Autodesk Inventor part; units mm, degrees
ref_plane "YZ Plane" through (0, 0, 0) normal (1, 0, 0) x (0, 1, 0)
ref_plane "XZ Plane" through (0, 0, 0) normal (0, 1, 0) x (-1, 0, 0)
ref_plane "XY Plane" through (0, 0, 0) normal (0, 0, 1) x (1, 0, 0)
sketch "Sketch1" plane through (0, 0, 0) normal (0, 1, 0) x (-1, 0, 0)
  line L0 (0, 0) -> (5.4973, 0)
  line L1 (5.4973, 0) -> (5.4973, -16.0791)
  line L2 (5.4973, -16.0791) -> (0, -16.0791)
  line L3 (0, -16.0791) -> (0, 0)
extrude "Extrusion1" add sketch "Sketch1" along normal blind 25.4
sketch "Sketch2" plane through (0, 0, 0) normal (1, 0, 0) x (0, 0, -1)
  line L0 (5.242, 8.6906) -> (11.0751, 8.6906)
  line L1 (11.0751, 8.6906) -> (11.0751, 5.3799)
  line L2 (11.0751, 5.3799) -> (5.242, 5.3799)
  line L3 (5.242, 5.3799) -> (5.242, 8.6906)
  line L4 (12.2594, 20.9027) -> (3.9371, 20.9027)
  line L5 (3.9371, 20.9027) -> (3.9371, 16.3797)
  line L6 (3.9371, 16.3797) -> (12.2594, 16.3797)
  line L7 (12.2594, 16.3797) -> (12.2594, 20.9027)
  point P0 (0, 0)
extrude "Extrusion2" add sketch "Sketch2" along normal blind 5
sketch "Sketch3" plane through (0, 25.4, 0) normal (0, 1, 0) x (1, 0, 0)
  point P0 (0, 0)
sketch "Sketch4" plane through (0, 16.3797, -12.2594) normal (0, 0, -1) x (-1, 0, 0)
  circle A0 centre (-2.546, 2.7504) radius 1.0051
  circle A1 centre (-2.546, -8.9893) radius 0.8063
  point P0 (0, -16.3797)
extrude "Extrusion3" add sketch "Sketch4" along normal blind 15 contours A0
sketch "Sketch5" plane through (0, 5.3799, -11.0751) normal (0, 0, -1) x (-1, 0, 0)
  circle A0 centre (-2.6874, 1.7983) radius 0.9619
  point P0 (0, -5.3799)
extrude "Extrusion4" add sketch "Sketch5" along normal blind 25
properties part number "niharika1"
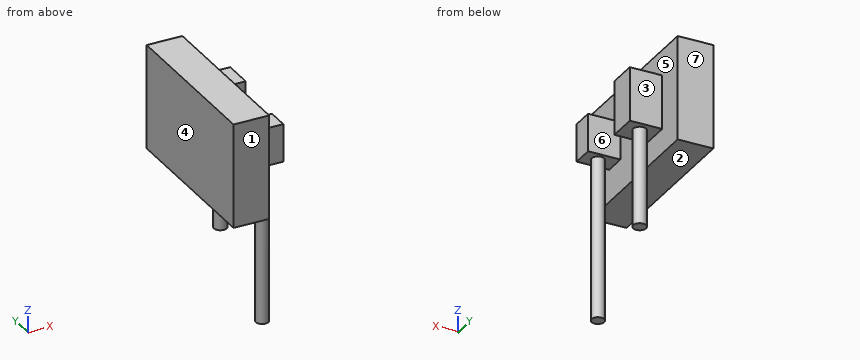
Verification items for the finished model (mm, model axes). Face numbers are marked on the shaded views. A direction names the side the tool comes from. Round coordinates to 2 decimals unless told otherwise and drop trailing zeros. Loops run counter-clockwise (first coordinate to the right, second up) from the corner with the lowest first, then second, coordinate; pieces in that order, holes last. Notation, with made-up numbers: (59, 72.25) -> (72, 72.25) arc R7 cw to (72, 80.25) -> close; hole circle Ø5 at (48.5, 55.25). An arc over 180 degrees is marked (long way). Answer as a JSON object with one key per item and string values.
Q1. Draft check along Y on the marked faces 4, 5, 6 and 7. Enter one of: pulls with the +Y half, pulls with the -Y half, needs draft (parallel to the pull), parting line crosses it, or undercut.
Data:
{"face 4": "needs draft", "face 5": "undercut", "face 6": "undercut", "face 7": "pulls with the +Y half"}
Q2. Section check D-D (x = -2.25). Record the boundary of the cut face in (y, z).
Data:
{"outline": "(0, -16.08) -> (25.4, -16.08) -> (25.4, 0) -> (0, 0) -> close"}
Q3. Go/stop test with flat-tipped pins: P1, Ø4, axis at x = 1, z = -26.5, coming from the -Y side; P2, Ø2.5, axis at x = 3, z = -8, coming from the +Y side; P3, Ø3.5, axis at x = 2, y = 18, coming from the +Z side; P4, Ø1.5, axis at x = -2.5, z = -10.5, coming from the -Y side. Record where each tip stops, or that it passes through.
Data:
{"P1": "stops at y = 6.22", "P2": "stops at y = 20.9", "P3": "stops at z = -3.94", "P4": "stops at y = 0"}
Q4. Access from +Z, -Z, +X, -X, +Y, -Y to the whole of each face (thin tool, end or side, straight path). Record for the marked faces 1, 2 and 3.
Data:
{"face 1": "+Z, -Z, +X, -X, -Y", "face 2": "-Z, -X, +Y, -Y", "face 3": "+Z, -Z, +X, +Y"}
Q5. Scan lines: line 1 (Y direction, x = 0.5, z = -12); line 2 (X direction, y = 12.25, z = -10.5); line 3 (Z direction, x = 0.25, y = 18.75). Record each from-to range of solid material in increasing order. Write a range as from..to.
Data:
{"line 1": "y = 16.38..20.9", "line 2": "x = -5.5..0", "line 3": "z = -12.26..-3.94"}
Q6. Section check A-A (x = 0.75). Record the boundary of the cut face in (y, z).
Data:
{"outline": "(5.38, -11.08) -> (8.69, -11.08) -> (8.69, -5.24) -> (5.38, -5.24) -> close; (16.38, -12.26) -> (20.9, -12.26) -> (20.9, -3.94) -> (16.38, -3.94) -> close"}
Q7. Section check B-B (z = -9). Record the boundary of the cut face in (x, y), then the cut area to 3 significant figures.
Data:
{"outline": "(-5.5, 0) -> (0, 0) -> (0, 5.38) -> (5, 5.38) -> (5, 8.69) -> (0, 8.69) -> (0, 16.38) -> (5, 16.38) -> (5, 20.9) -> (0, 20.9) -> (0, 25.4) -> (-5.5, 25.4) -> close", "area": "179 mm2"}
Q8. Section check C-C (z = -13). Record the boundary of the cut face in (x, y).
Data:
{"outline": "(-5.5, 0) -> (0, 0) -> (0, 25.4) -> (-5.5, 25.4) -> close; circle Ø2.01 at (2.55, 19.13); circle Ø1.92 at (2.69, 7.18)"}
